Can you work these out from the model? Positions are in its coordinate system, mm. Face numbers are marked on the shaded views. Give positions to 0.01 mm unless a question says otherwise; leave off trailing zeros. Write each loop counter-clockwise with the first axis right and the second up, starting at its lowest first coordinate (ties: lowest second). Pieces come first, ordered by that corner, then holes.
from build123d import *

# Parameters (mm, degrees)
SKETCH1_R             = 1.6
BOSS_EXTRUDE1_DEPTH   = 30
BOSS_EXTRUDE1_2_DEPTH = 30
BOSS_EXTRUDE1_3_DEPTH = 30
BOSS_EXTRUDE1_4_DEPTH = 30
BOSS_EXTRUDE2_DEPTH   = 3
SKETCH3_R             = 1.75
CUT_EXTRUDE1_DEPTH    = 3


with BuildPart() as part:
    # Sketch1 → Boss-Extrude1 (new body)
    with BuildSketch(Plane(origin=(0, 0, 0), x_dir=(1, 0, 0), z_dir=(0, 1, 0))):
        with BuildLine():
            Line((-1.25, 4.658509183), (-3.033431688, 2.204720435))
            ThreePointArc((-3.033431688, 2.204720435), (-3.75, 0), (-3.033431688, -2.204720435))
            Line((-3.033431688, -2.204720435), (-1.25, -4.658509183))
            ThreePointArc((-1.25, -4.658509183), (0, -5.295279565), (1.25, -4.658509183))
            Line((1.25, -4.658509183), (3.033431688, -2.204720435))
            ThreePointArc((3.033431688, -2.204720435), (3.75, 0), (3.033431688, 2.204720435))
            Line((3.033431688, 2.204720435), (1.25, 4.658509183))
            ThreePointArc((1.25, 4.658509183), (0, 5.295279565), (-1.25, 4.658509183))
        make_face()
        with Locations(Location((0, 0, 0), (0, 0, 270))):
            Circle(SKETCH1_R, mode=Mode.SUBTRACT)
    extrude(amount=BOSS_EXTRUDE1_DEPTH)



with BuildPart() as body_2:
    # Sketch1 → Boss-Extrude1 2 (new body)
    with BuildSketch(Plane(origin=(0, 0, 0), x_dir=(1, 0, 0), z_dir=(0, 1, 0))):
        with BuildLine():
            Line((68.75, 4.658509183), (66.966568312, 2.204720435))
            ThreePointArc((66.966568312, 2.204720435), (66.25, 0), (66.966568312, -2.204720435))
            Line((66.966568312, -2.204720435), (68.75, -4.658509183))
            ThreePointArc((68.75, -4.658509183), (70, -5.295279565), (71.25, -4.658509183))
            Line((71.25, -4.658509183), (73.033431688, -2.204720435))
            ThreePointArc((73.033431688, -2.204720435), (73.75, 0), (73.033431688, 2.204720435))
            Line((73.033431688, 2.204720435), (71.25, 4.658509183))
            ThreePointArc((71.25, 4.658509183), (70, 5.295279565), (68.75, 4.658509183))
        make_face()
        with Locations(Location((70, 0, 0), (0, 0, 270))):
            Circle(SKETCH1_R, mode=Mode.SUBTRACT)
    extrude(amount=BOSS_EXTRUDE1_2_DEPTH)


with BuildPart() as body_3:
    # Sketch1 → Boss-Extrude1 3 (new body)
    with BuildSketch(Plane(origin=(0, 0, 0), x_dir=(1, 0, 0), z_dir=(0, 1, 0))):
        with BuildLine():
            Line((68.75, -35.341490817), (66.966568312, -37.795279565))
            ThreePointArc((66.966568312, -37.795279565), (66.25, -40), (66.966568312, -42.204720435))
            Line((66.966568312, -42.204720435), (68.75, -44.658509183))
            ThreePointArc((68.75, -44.658509183), (70, -45.295279565), (71.25, -44.658509183))
            Line((71.25, -44.658509183), (73.033431688, -42.204720435))
            ThreePointArc((73.033431688, -42.204720435), (73.75, -40), (73.033431688, -37.795279565))
            Line((73.033431688, -37.795279565), (71.25, -35.341490817))
            ThreePointArc((71.25, -35.341490817), (70, -34.704720435), (68.75, -35.341490817))
        make_face()
        with Locations(Location((70, -40, 0), (0, 0, 270))):
            Circle(SKETCH1_R, mode=Mode.SUBTRACT)
    extrude(amount=BOSS_EXTRUDE1_3_DEPTH)


with BuildPart() as body_4:
    # Sketch1 → Boss-Extrude1 4 (new body)
    with BuildSketch(Plane(origin=(0, 0, 0), x_dir=(1, 0, 0), z_dir=(0, 1, 0))):
        with BuildLine():
            Line((-1.25, -35.341490817), (-3.033431688, -37.795279565))
            ThreePointArc((-3.033431688, -37.795279565), (-3.75, -40), (-3.033431688, -42.204720435))
            Line((-3.033431688, -42.204720435), (-1.25, -44.658509183))
            ThreePointArc((-1.25, -44.658509183), (0, -45.295279565), (1.25, -44.658509183))
            Line((1.25, -44.658509183), (3.033431688, -42.204720435))
            ThreePointArc((3.033431688, -42.204720435), (3.75, -40), (3.033431688, -37.795279565))
            Line((3.033431688, -37.795279565), (1.25, -35.341490817))
            ThreePointArc((1.25, -35.341490817), (0, -34.704720435), (-1.25, -35.341490817))
        make_face()
        with Locations(Location((0, -40, 0), (0, 0, 270))):
            Circle(SKETCH1_R, mode=Mode.SUBTRACT)
    extrude(amount=BOSS_EXTRUDE1_4_DEPTH)


with BuildPart() as part_1:
    add(part.part)

    add(body_2.part)  # Boss-Extrude2 merges body 2

    add(body_3.part)  # Boss-Extrude2 merges body 3

    add(body_4.part)  # Boss-Extrude2 merges body 4
    # Sketch2 → Boss-Extrude2 (add)
    with BuildSketch(Plane(origin=(0, 30, 0), x_dir=(1, 0, 0), z_dir=(0, 1, 0))):
        with BuildLine():
            Line((-3.75, 0), (-3.75, -40))
            ThreePointArc((-3.75, -40), (-3.566361509, -41.159122765), (-3.033431688, -42.204720435))
            Line((-3.033431688, -42.204720435), (-1.25, -44.658509183))
            ThreePointArc((-1.25, -44.658509183), (-0.701422932, -45.126914959), (0, -45.295279565))
            Line((0, -45.295279565), (70, -45.295279565))
            ThreePointArc((70, -45.295279565), (70.701422932, -45.126914959), (71.25, -44.658509183))
            Line((71.25, -44.658509183), (73.033431688, -42.204720435))
            ThreePointArc((73.033431688, -42.204720435), (73.566361509, -41.159122765), (73.75, -40))
            Line((73.75, -40), (73.75, 0))
            ThreePointArc((73.75, 0), (73.566361509, 1.159122765), (73.033431688, 2.204720435))
            Line((73.033431688, 2.204720435), (71.25, 4.658509183))
            ThreePointArc((71.25, 4.658509183), (70.701422932, 5.126914959), (70, 5.295279565))
            Line((70, 5.295279565), (0, 5.295279565))
            ThreePointArc((0, 5.295279565), (-0.701422932, 5.126914959), (-1.25, 4.658509183))
            Line((-1.25, 4.658509183), (-3.033431688, 2.204720435))
            ThreePointArc((-3.033431688, 2.204720435), (-3.566361509, 1.159122765), (-3.75, 0))
        make_face()
        with BuildLine():
            Line((8.75, -34.704720435), (61.25, -34.704720435))
            ThreePointArc((61.25, -34.704720435), (64.785533906, -33.240254341), (66.25, -29.704720435))
            Line((66.25, -29.704720435), (66.25, -10.295279565))
            ThreePointArc((66.25, -10.295279565), (64.785533906, -6.759745659), (61.25, -5.295279565))
            Line((61.25, -5.295279565), (8.75, -5.295279565))
            ThreePointArc((8.75, -5.295279565), (5.214466094, -6.759745659), (3.75, -10.295279565))
            Line((3.75, -10.295279565), (3.75, -29.704720435))
            ThreePointArc((3.75, -29.704720435), (5.214466094, -33.240254341), (8.75, -34.704720435))
        make_face(mode=Mode.SUBTRACT)
    extrude(amount=BOSS_EXTRUDE2_DEPTH)

    # Sketch3 → Cut-Extrude1 (cut)
    with BuildSketch(Plane(origin=(0, 33, 0), x_dir=(1, 0, 0), z_dir=(0, 1, 0))):
        with Locations(Location((35, -0.004720435, 0), (0, 0, 270))):
            Circle(SKETCH3_R)
        with Locations(Location((35, -40.004720435, 0), (0, 0, 270))):
            Circle(SKETCH3_R)
    extrude(amount=-CUT_EXTRUDE1_DEPTH, mode=Mode.SUBTRACT)


solid = part_1.part
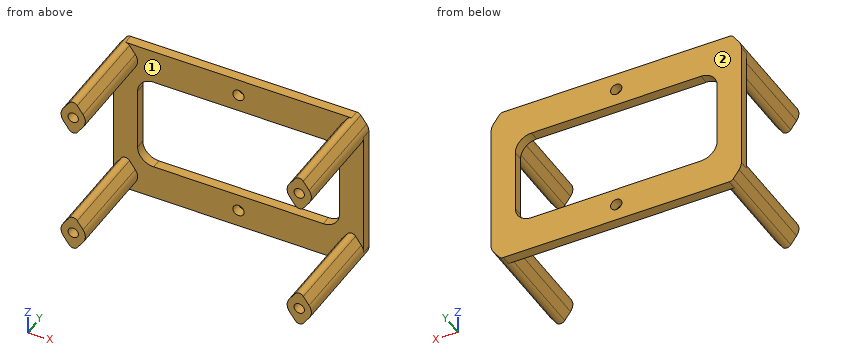
(1) Imagine slicing it at C-C, the plane x = 10.5. Write out the boundary of the cut face in (y, z).
Returned:
outline: (30, -5.3) - (33, -5.3) - (33, 5.3) - (30, 5.3) - close; (30, 34.7) - (33, 34.7) - (33, 45.3) - (30, 45.3) - close
(2) If I drill on L1, parallel to Z at x = 70, y = 10; L2, parallel to X at y = 12, z = 0; L3, parallel to Y at x = 12.5, z = 38, over which ranges is the centre line in solid material (lowest first)?
Returned:
L1: z = -5.3 to -1.6, 1.6 to 5.3, 34.7 to 38.4, 41.6 to 45.3
L2: x = -3.75 to -1.6, 1.6 to 3.75, 66.25 to 68.4, 71.6 to 73.75
L3: y = 30 to 33
(3) Will these pins go through, and if not, where does the flat tip stop? P1, Ø2, axis at x = 35.5, z = 38.5, coming from the -Y side; P2, Ø1, axis at y = 27, z = 35.5, coming from the -X side; P3, Ø12, axis at y = 4, z = 27.5, coming from the +X side; P4, Ø1.5, axis at y = 20, z = 35.5, coming from the -X side.
Returned:
P1: stops at y = 30
P2: stops at x = -1.73
P3: passes through
P4: stops at x = -1.91
(4) Imagine slicing it at B-B, the plane z = 13.5. Write out the boundary of the cut face in (x, y), plus the area to 3 significant figures.
Returned:
outline: (-3.75, 30) - (3.75, 30) - (3.75, 33) - (-3.75, 33) - close; (66.25, 30) - (73.75, 30) - (73.75, 33) - (66.25, 33) - close
area: 45.0 mm2
(5) Imagine slicing it at A-A, the plane x = 35. Write out the boundary of the cut face in (y, z), plus the area to 3 significant figures.
Returned:
outline: (30, -5.3) - (33, -5.3) - (33, -1.75) - (30, -1.75) - close; (30, 1.75) - (33, 1.75) - (33, 5.3) - (30, 5.3) - close; (30, 34.7) - (33, 34.7) - (33, 38.25) - (30, 38.25) - close; (30, 41.75) - (33, 41.75) - (33, 45.3) - (30, 45.3) - close
area: 42.5 mm2
(6) Imagine slicing it at D-D, the plane y = 26. Give the number of separate pieces and of enclosed holes in the cut face, plus the area to 3 significant figures.
Returned:
separate pieces: 4
enclosed holes: 4
area: 185 mm2
(7) If we mould it in two halves opening along Z, with no side actions, what happens to the marked faces 1 and 2? For each: +Z half, -Z half, draft (parallel to the pull), parting line (faces both ways), or undercut.
Returned:
face 1: undercut
face 2: draft
